Geometry check sheet. Reference: drawing and pictorial views, mm from the part's lowest x, y, z. A direction names the side the tool comes from. Coordinates: 2 decimals unless noted, no trailing zeros. Write each loop counter-clockwise with the first axis right and the second up, starting at its lowest first coordinate (ties: lowest second). Pieces come first, ordered by that corner, then holes. Notation, with made-up numbers: (-34.75, 63) -> (13.25, 63) arc R19 cw to (13.25, 93) -> close; hole circle Ø4 at (77, 5.25). An arc over 180 degrees is marked (long way). Answer in a Markdown table with one row per item.
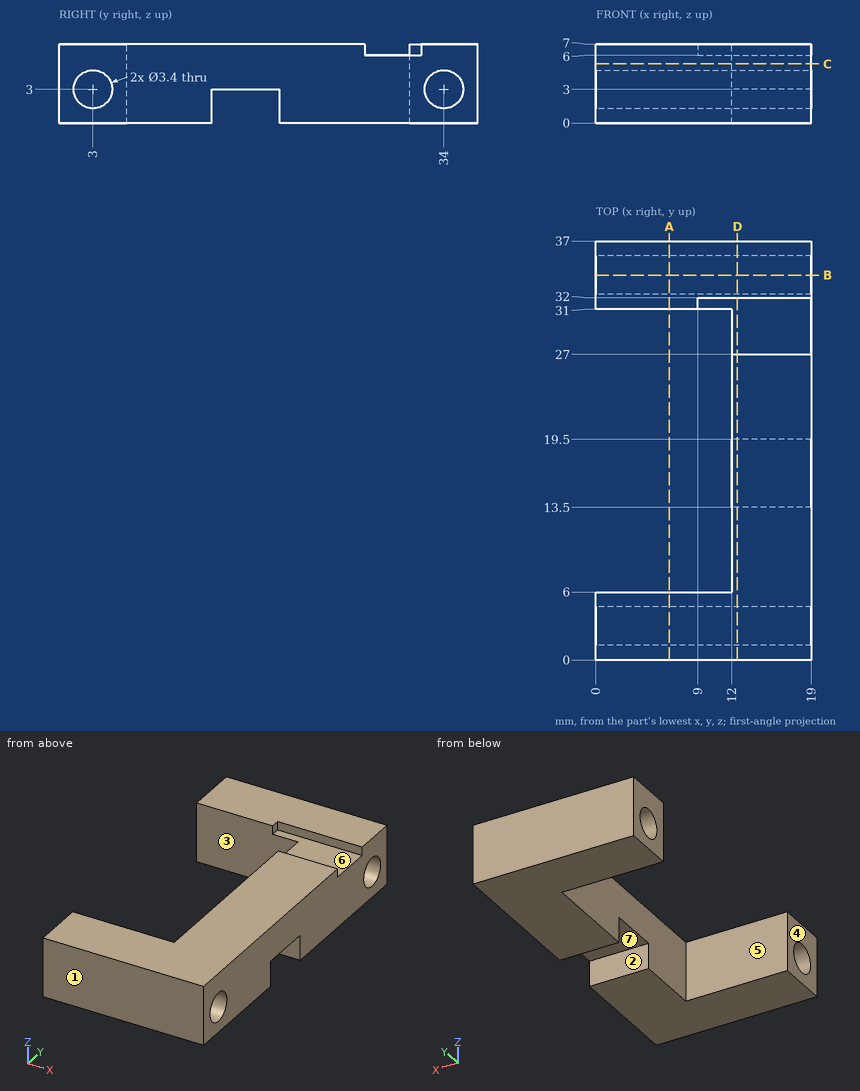
1. Mould release check, pull along Y, two halves, no side actions. Record for the marked faces 1, 2, 3 and 4: released by +Y, released by -Y, zero draft, split by the parting line, or undercut.
Geometry says:
| item | result |
|---|---|
| face 1 | released by -Y |
| face 2 | undercut |
| face 3 | undercut |
| face 4 | zero draft |
2. Section check B-B, the plane y = 34. Record the boundary of the cut face in (x, z).
Geometry says:
| item | result |
|---|---|
| outline | (0, 0) -> (19, 0) -> (19, 1.3) -> (0, 1.3) -> close; (0, 4.7) -> (19, 4.7) -> (19, 7) -> (0, 7) -> close |
3. Section check D-D, the plane x = 12.5. Record the boundary of the cut face in (y, z), plus the area to 3 significant figures.
Geometry says:
| item | result |
|---|---|
| outline | (0, 0) -> (13.5, 0) -> (13.5, 3) -> (19.5, 3) -> (19.5, 0) -> (37, 0) -> (37, 7) -> (32, 7) -> (32, 6) -> (27, 6) -> (27, 7) -> (0, 7) -> close; hole circle Ø3.4 at (3, 3); hole circle Ø3.4 at (34, 3) |
| area | 218 mm^2 |
4. Depth check by flat-ended pin: P1, Ø1.5, axis at x = 12, y = 30.5, coming from the +Z side; P2, Ø2, axis at y = 24.5, z = 4, coming from the -X side; P3, Ø0.8, axis at y = 31.5, z = 6.5, coming from the +X side. Enter the tip coordinate at first touch or a pass-through.
Geometry says:
| item | result |
|---|---|
| P1 | z = 6 |
| P2 | x = 12 |
| P3 | x = 9 |
5. Tool access check on the marked faces 5, 6 and 7. Record the directions out of +Z, -Z, +X, -X, +Y, -Y that give a thin tool (end or side, any length) a straight path to the whole face; none if there is none.
Geometry says:
| item | result |
|---|---|
| face 5 | +Z, -Z, -X |
| face 6 | +Z, +X |
| face 7 | -Z, +X, -X |
6. Section check C-C, the plane z = 5.25. Record the boundary of the cut face in (x, y), plus the area to 3 significant figures.
Geometry says:
| item | result |
|---|---|
| outline | (0, 0) -> (19, 0) -> (19, 37) -> (0, 37) -> (0, 31) -> (12, 31) -> (12, 6) -> (0, 6) -> close |
| area | 403 mm^2 |
7. Thickness scan on line 1 (Y direction, x = 5.75, z = 3); line 2 (Y direction, x = 17.25, z = 2.25); line 3 (Y direction, x = 11.25, z = 0.5). Record the ranges inside material, lowest first. Write a range as from..to.
Geometry says:
| item | result |
|---|---|
| line 1 | 0..1.3, 4.7..6, 31..32.3, 35.7..37 |
| line 2 | 0..1.47, 4.53..13.5, 19.5..32.47, 35.53..37 |
| line 3 | 0..6, 31..37 |
8. Section check A-A, the plane x = 6.5. Record the boundary of the cut face in (y, z).
Geometry says:
| item | result |
|---|---|
| outline | (0, 0) -> (6, 0) -> (6, 7) -> (0, 7) -> close; (31, 0) -> (37, 0) -> (37, 7) -> (31, 7) -> close; hole circle Ø3.4 at (3, 3); hole circle Ø3.4 at (34, 3) |
